Read the model definition and answer for the solid it produces. Units are mm, in the model's axes. A direction names the side the tool comes from. Give positions to 0.01 mm unless a question says otherwise; leave off trailing zeros. Order: outer loops, then holes, each group sorted by start corner. A loop starts at its lowest first (then second) coordinate and runs counter-clockwise, first axis right, second up.
Item 1: A cutting plane is placed at B-B (y = -21). Write down the section's boundary in (x, z), plus the area to 3 significant figures.
Item 2: Which of the six approach directions +Z, -Z, +X, -X, +Y, -Y give full straight-line access (tool end or side, diameter ignored) to faces 4 (the face through (-92, -22, -44)), 5 (the face through (49.21, 77.524, -49.336)), 6 (the face through (-102, -8, -44))?
Item 3: Find the intervals of material crossed by line 1 along X through (y, z) = (-29, -20); line 2 along Z through (x, y) = (41, 58); line 3 along X through (y, z) = (-12, -4), in increasing order.
Item 4: A cutting plane is placed at A-A (x = -129). Write down the section's boundary in (y, z), plus the area to 3 significant figures.
Item 5: Given pin 1 Ø1.5 at (y, z) = (51, -58) entering from -X; pin 2 Ø5 at (x, z) = (-14, -68.5) entering from +Y; pin 3 Ø10 at (x, z) = (-62, -74) entering from +Y; pin 4 Ø16 at (y, z) = (58, -45) entering from -X, each flat-ended and moving along its own axis, determine where each tip first touches the part or whether it passes through.
Item 6: A cutting plane is placed at C-C (y = 51.5). State how many separate pieces and enclosed holes the cut face has, plus the area to 3 significant figures.
Item 7: The mould has two halves that part along Z. Classify faces 1 (the face through (-44, 33, -46)), 2 (the face through (-2, 2, -90)), 3 (the face through (-133.73, -29.93, -64.84)): +Z half, -Z half, draft (parallel to the pull), parting line (faces both ways), or undercut.
from build123d import *

# Parameters (mm, degrees)
BOSS_EXTRUDE1_DEPTH      = 90
FILLET1_R                = 10
SKETCH2_R                = 7
CUT_EXTRUDE1_DEPTH       = 10
SKETCH10_R               = 20
SKETCH10_R_2             = 10
BOSS_EXTRUDE5_DEPTH      = 68
SKETCH11_R               = 20
SKETCH11_R_2             = 10
CUT_EXTRUDE5_DEPTH       = 38
BOSS_EXTRUDE6_DEPTH      = 5
BOSS_EXTRUDE6_DEPTH_BACK = 5
FILLET3_R                = 10
SKETCH15_R               = 20
SKETCH15_R_2             = 10
BOSS_EXTRUDE7_DEPTH      = 68
CUT_EXTRUDE6_START       = -38
SKETCH16_R               = 20
SKETCH16_R_2             = 10
CUT_EXTRUDE6_DEPTH       = 38
BOSS_EXTRUDE8_DEPTH      = 5
BOSS_EXTRUDE8_DEPTH_BACK = 5
FILLET4_R                = 10


with BuildPart() as part:
    # Sketch1 → Boss-Extrude1 (new body)
    with BuildSketch(Plane.XY):
        Polygon((-102, 10), (102, 10), (102, -25), (146, -25), (146, -35), (92, -35), (92, 0), (-92, 0), (-92, -35), (-146, -35), (-146, -25), (-102, -25), align=None)
    extrude(amount=-BOSS_EXTRUDE1_DEPTH)

    # Fillet1
    fillet1_edges = [part.edges().sort_by_distance(p)[0] for p in [
        (-102, -25, -45),
        (-102, 10, -45),
        (102, 10, -45),
        (102, -25, -45),
    ]]
    fillet(fillet1_edges, radius=FILLET1_R)

    # Sketch2 → Cut-Extrude1 (cut)
    with BuildSketch(Plane(origin=(0, -25, 0), x_dir=(1, 0, 0), z_dir=(0, 1, 0))):
        with Locations(Location((129, 20, 0), (0, 0, 270))):
            Circle(SKETCH2_R)
        with Locations(Location((129, 70, 0), (0, 0, 270))):
            Circle(SKETCH2_R)
        with Locations(Location((-129, 70, 0), (0, 0, 90))):
            Circle(SKETCH2_R)
        with Locations(Location((-129, 20, 0), (0, 0, 90))):
            Circle(SKETCH2_R)
    extrude(amount=-CUT_EXTRUDE1_DEPTH, mode=Mode.SUBTRACT)



with BuildPart() as body_2:
    # Sketch10 → Boss-Extrude5 (new body)
    with BuildSketch(Plane.ZY.offset(102)):
        with Locations((-45, 48)):
            Circle(SKETCH10_R)
        with Locations((-45, 48)):
            Circle(SKETCH10_R_2, mode=Mode.SUBTRACT)
    extrude(amount=-BOSS_EXTRUDE5_DEPTH)

    # Sketch11 → Cut-Extrude5 (cut)
    with BuildSketch(Plane.ZY.offset(102)):
        with Locations((-45, 48)):
            Circle(SKETCH11_R)
        with Locations((-45, 48)):
            Circle(SKETCH11_R_2, mode=Mode.SUBTRACT)
    extrude(amount=-CUT_EXTRUDE5_DEPTH, mode=Mode.SUBTRACT)


with BuildPart() as body_2_1:
    # Body-Move/Copy1: moved
    add(body_2.part.moved(Location((0, 10, 0))))


with BuildPart() as part_1:
    add(part.part)

    add(body_2_1.part)  # Boss-Extrude6 merges body 2
    # Sketch14 → Boss-Extrude6 (add, two sides: drawn at the far end of the back side and taken through both)
    with BuildSketch(Plane(origin=(-49, 0, 0), x_dir=(0, 0, -1), z_dir=(1, 0, 0)).offset(-BOSS_EXTRUDE6_DEPTH_BACK)):
        with BuildLine():
            Line((45, 10), (0, 10))
            Line((0, 10), (26.941680216, 66.596341464))
            ThreePointArc((26.941680216, 66.596341464), (45, 38), (63.058319784, 66.596341464))
            Line((63.058319784, 66.596341464), (90, 10))
            Line((90, 10), (45, 10))
        make_face()
    extrude(amount=BOSS_EXTRUDE6_DEPTH + BOSS_EXTRUDE6_DEPTH_BACK)

    # Fillet3
    # the kernel refuses this fillet: 10 mm, written as the material it adds along each edge
    with BuildSketch(Plane(origin=(-54, 10, 0), x_dir=(-1, 0, 0), z_dir=(0, 0, -1))) as fillet3_piece_1_section:
        with BuildLine():
            CenterArc((FILLET3_R, FILLET3_R), FILLET3_R, 180, 90)
            Line((0, FILLET3_R), (0, 0))
            Line((0, 0), (FILLET3_R, 0))
        make_face()
    fillet3_piece_1 = extrude(amount=90, mode=Mode.PRIVATE)
    fillet3_piece_1 = split(fillet3_piece_1, bisect_by=Plane(origin=(-56.293482883, 29.268794576, -9.172566427), z_dir=(0, -0.4298170732175253, -0.9029159892098049)), keep=Keep.TOP, mode=Mode.PRIVATE)
    fillet3_piece_1 = split(fillet3_piece_1, bisect_by=Plane(origin=(-56.293482883, 29.268794576, -80.827433573), z_dir=(0, -0.4298170732175253, 0.9029159892098049)), keep=Keep.TOP, mode=Mode.PRIVATE)
    add(fillet3_piece_1)
    with BuildSketch(Plane(origin=(-44, 10, -90), x_dir=(1, 0, 0), z_dir=(0, 0, 1))) as fillet3_piece_2_section:
        with BuildLine():
            CenterArc((FILLET3_R, FILLET3_R), FILLET3_R, 180, 90)
            Line((0, FILLET3_R), (0, 0))
            Line((0, 0), (FILLET3_R, 0))
        make_face()
    fillet3_piece_2 = extrude(amount=90, mode=Mode.PRIVATE)
    fillet3_piece_2 = split(fillet3_piece_2, bisect_by=Plane(origin=(-41.706517117, 29.268794576, -9.172566427), z_dir=(0, -0.4298170732175253, -0.9029159892098049)), keep=Keep.TOP, mode=Mode.PRIVATE)
    fillet3_piece_2 = split(fillet3_piece_2, bisect_by=Plane(origin=(-41.706517117, 29.268794576, -80.827433573), z_dir=(0, -0.4298170732175253, 0.9029159892098049)), keep=Keep.TOP, mode=Mode.PRIVATE)
    add(fillet3_piece_2)



with BuildPart() as body_2_2:
    # Sketch15 → Boss-Extrude7 (new body)
    with BuildSketch(Plane(origin=(102, 0, 0), x_dir=(0, 0, -1), z_dir=(1, 0, 0))):
        with Locations(Location((45, 58, 0), (0, 0, 180))):
            Circle(SKETCH15_R)
        with Locations(Location((45, 58, 0), (0, 0, 180))):
            Circle(SKETCH15_R_2, mode=Mode.SUBTRACT)
    extrude(amount=-BOSS_EXTRUDE7_DEPTH)

    # Sketch16 → Cut-Extrude6 (cut)
    with BuildSketch(Plane(origin=(102, 0, 0), x_dir=(0, 0, -1), z_dir=(1, 0, 0)).offset(CUT_EXTRUDE6_START)):
        with Locations(Location((45, 58, 0), (0, 0, 180))):
            Circle(SKETCH16_R)
        with Locations(Location((45, 58, 0), (0, 0, 180))):
            Circle(SKETCH16_R_2, mode=Mode.SUBTRACT)
    extrude(amount=CUT_EXTRUDE6_DEPTH, mode=Mode.SUBTRACT)


with BuildPart() as part_2:
    add(part_1.part)

    add(body_2_2.part)  # Boss-Extrude8 merges body 2 2
    # Sketch17 → Boss-Extrude8 (add, two sides: drawn at the far end of the back side and taken through both)
    with BuildSketch(Plane(origin=(49, 0, 0), x_dir=(0, 0, -1), z_dir=(1, 0, 0)).offset(-BOSS_EXTRUDE8_DEPTH_BACK)):
        with BuildLine():
            Line((45, 10), (0, 10))
            Line((0, 10), (26.941680216, 66.596341464))
            ThreePointArc((26.941680216, 66.596341464), (45, 38), (63.058319784, 66.596341464))
            Line((63.058319784, 66.596341464), (90, 10))
            Line((90, 10), (45, 10))
        make_face()
    extrude(amount=BOSS_EXTRUDE8_DEPTH + BOSS_EXTRUDE8_DEPTH_BACK)

    # Fillet4
    # the kernel refuses this fillet: 10 mm, written as the material it adds along each edge
    with BuildSketch(Plane(origin=(44, 10, 0), x_dir=(-1, 0, 0), z_dir=(0, 0, -1))) as fillet4_piece_1_section:
        with BuildLine():
            CenterArc((FILLET4_R, FILLET4_R), FILLET4_R, 180, 90)
            Line((0, FILLET4_R), (0, 0))
            Line((0, 0), (FILLET4_R, 0))
        make_face()
    fillet4_piece_1 = extrude(amount=90, mode=Mode.PRIVATE)
    fillet4_piece_1 = split(fillet4_piece_1, bisect_by=Plane(origin=(41.706517117, 29.268794576, -80.827433573), z_dir=(0, -0.4298170732175253, 0.9029159892098049)), keep=Keep.TOP, mode=Mode.PRIVATE)
    fillet4_piece_1 = split(fillet4_piece_1, bisect_by=Plane(origin=(41.706517117, 29.268794576, -9.172566427), z_dir=(0, -0.4298170732175254, -0.9029159892098049)), keep=Keep.TOP, mode=Mode.PRIVATE)
    add(fillet4_piece_1)
    with BuildSketch(Plane(origin=(54, 10, -90), x_dir=(1, 0, 0), z_dir=(0, 0, 1))) as fillet4_piece_2_section:
        with BuildLine():
            CenterArc((FILLET4_R, FILLET4_R), FILLET4_R, 180, 90)
            Line((0, FILLET4_R), (0, 0))
            Line((0, 0), (FILLET4_R, 0))
        make_face()
    fillet4_piece_2 = extrude(amount=90, mode=Mode.PRIVATE)
    fillet4_piece_2 = split(fillet4_piece_2, bisect_by=Plane(origin=(56.293482883, 29.268794576, -9.172566427), z_dir=(0, -0.4298170732175254, -0.9029159892098049)), keep=Keep.TOP, mode=Mode.PRIVATE)
    fillet4_piece_2 = split(fillet4_piece_2, bisect_by=Plane(origin=(56.293482883, 29.268794576, -80.827433573), z_dir=(0, -0.4298170732175253, 0.9029159892098049)), keep=Keep.TOP, mode=Mode.PRIVATE)
    add(fillet4_piece_2)
    with BuildSketch(Plane(origin=(92, 0, 0), x_dir=(0, -1, 0), z_dir=(0, 0, -1)), Plane(origin=(-92, 0, 0), x_dir=(1, 0, 0), z_dir=(0, 0, -1))) as fillet4_piece_3:
        with BuildLine():
            CenterArc((FILLET4_R, FILLET4_R), FILLET4_R, 180, 90)
            Line((0, FILLET4_R), (0, 0))
            Line((0, 0), (FILLET4_R, 0))
        make_face()
    extrude(amount=90)


solid = part_2.part
Response values:
1. outline: (-104, -90) - (-92, -90) - (-92, 0) - (-104, 0) - close; (92, -90) - (104, -90) - (104, 0) - (92, 0) - close
1. area: 2,160 mm2
2. face 4: +Z, -Z, -Y
2. face 5: none
2. face 6: +Z, -Z, -X, +Y
3. line 1: x = -146 to -136, -122 to -92, 92 to 122, 136 to 146
3. line 2: z = -65 to -55, -35 to -25
3. line 3: x = -102 to -92, 92 to 102
4. outline: (-35, -90) - (-25, -90) - (-25, -77) - (-35, -77) - close; (-35, -63) - (-25, -63) - (-25, -27) - (-35, -27) - close; (-35, -13) - (-25, -13) - (-25, 0) - (-35, 0) - close
4. area: 620 mm2
5. pin 1: stops at x = -64
5. pin 2: stops at y = 10
5. pin 3: stops at y = 12.86
5. pin 4: passes through
6. separate pieces: 4
6. enclosed holes: 0
6. area: 1,610 mm2
7. face 1: draft
7. face 2: -Z half
7. face 3: undercut
